For this review, use the dimensioned drawing (mm, ordinates from the lowest corner) and the shaded views. A direction names the side the tool comes from. Give positions to 0.01 mm unless a question says otherwise; leave off trailing zeros. Order: outer loops, then holes, each group sorted by start corner. A loop starts at its lowest first (then second) coordinate and runs counter-clockwise, first axis right, second up.
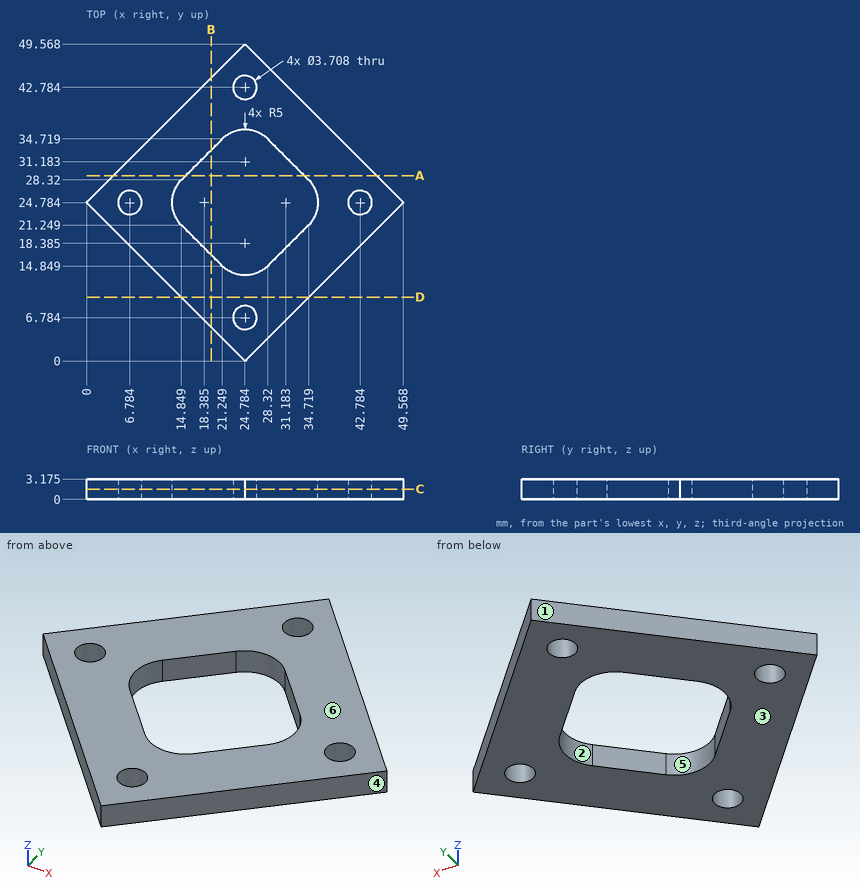
1. Take a section at B-B (x = 19.5). State the section outline as (y, z) points (1 decimal).
Recorded:
outline: (5.3, 0) - (16.6, 0) - (16.6, 3.2) - (5.3, 3.2) - close; (33, 0) - (44.3, 0) - (44.3, 3.2) - (33, 3.2) - close
2. Draft analysis for pull direction X (two halves, no side actions). For the marked faces 1, 2, 3 and 4, state which applies: pulls with the +X half, pulls with the -X half, needs draft (parallel to the pull), parting line crosses it, or undercut.
Recorded:
face 1: pulls with the -X half
face 2: undercut
face 3: needs draft
face 4: pulls with the +X half
3. Take a section at D-D (y = 10). State the section outline as (x, z) points (1 decimal).
Recorded:
outline: (14.8, 0) - (34.8, 0) - (34.8, 3.2) - (14.8, 3.2) - close
4. For line 1 along X through (y, z) = (21, 0.9) (1 decimal); line 2 along X through (y, z) = (6, 2.85) (1 decimal); line 3 along Y through (x, z) = (18, 2.65) (1 decimal), list the stretches that pass through material, from the lowest coordinate up.
Recorded:
line 1: x = 3.8 to 15.1, 34.5 to 45.8
line 2: x = 18.8 to 23.1, 26.5 to 30.8
line 3: y = 6.8 to 18.1, 31.5 to 42.8
5. For pin 1 (1.5 mm diameter, centred on x = 15, z = 1.5, fed in from +Y) (1 decimal), flat-tipped, find the tip position at first contact; note if it passes through.
Recorded:
pin 1: stops at y = 40.5
6. Machinability: for the marked faces 5 and 6, which of the approach directions +Z, -Z, +X, -X, +Y, -Y give a long, thin tool a straight path to every point of the face, cutting with its end or side? Answer none if there is none.
Recorded:
face 5: +Z, -Z
face 6: +Z, +X, -X, +Y, -Y
7. Take a section at A-A (y = 29). State the section outline as (x, z) points (1 decimal).
Recorded:
outline: (4.2, 0) - (15.5, 0) - (15.5, 3.2) - (4.2, 3.2) - close; (34, 0) - (45.4, 0) - (45.4, 3.2) - (34, 3.2) - close
8. Take a section at C-C (z = 1.6). State how many separate pieces and enclosed holes the cut face has, then the cut area to 3 significant figures.
Recorded:
separate pieces: 1
enclosed holes: 5
area: 844 mm2
